```python
from build123d import *

# Parameters (mm, degrees)
CROQUIS1_R                = 1.5
SALIENTE_EXTRUIR2_DEPTH   = 3
SALIENTE_EXTRUIR2_2_DEPTH = 3
SALIENTE_EXTRUIR3_DEPTH   = 3
CROQUIS4_R                = 1.5
CORTAR_EXTRUIR2_DEPTH     = 3
SALIENTE_EXTRUIR4_START   = -3
CROQUIS5_R                = 1.5
SALIENTE_EXTRUIR4_DEPTH   = 3
SALIENTE_EXTRUIR5_DEPTH   = 15
CROQUIS7_R                = 1.5
CORTAR_EXTRUIR3_DEPTH     = 15
CROQUIS8_R                = 1.5
CORTAR_EXTRUIR4_DEPTH     = 15
CROQUIS9_R                = 1.5
CORTAR_EXTRUIR5_DEPTH     = 15
CROQUIS10_W               = 207.078994109
CROQUIS10_H               = 142.865408101
CORTAR_EXTRUIR6_DEPTH     = 20
SALIENTE_EXTRUIR6_DEPTH   = 3
CORTAR_EXTRUIR9_DEPTH     = 6
SALIENTE_EXTRUIR8_DEPTH   = 6
CROQUIS14_W               = 35.322230026
CROQUIS14_H               = 29.345994137
CORTAR_EXTRUIR10_DEPTH    = 3
CROQUIS15_W               = 36.043333432
CROQUIS15_H               = 18.319096506
CORTAR_EXTRUIR12_DEPTH    = 10
SALIENTE_EXTRUIR9_DEPTH   = 15
CROQUIS17_R               = 1.5
CORTAR_EXTRUIR14_DEPTH    = 30
CROQUIS18_R               = 1.5
CORTAR_EXTRUIR15_DEPTH    = 30


with BuildPart() as part:
    # Croquis1 → Saliente-Extruir2 (new body)
    with BuildSketch(Plane(origin=(0, 0, 0), x_dir=(1, 0, 0), z_dir=(0, 1, 0))):
        Polygon((35, 0), (65, 0), (167.530483272, -102.530483272), (161.873629023, -108.187337522), (61.686291501, -8), (35, -8), align=None)
        with Locations(Location((50, -4, 0), (0, 0, 270))):
            Circle(CROQUIS1_R, mode=Mode.SUBTRACT)
        with Locations(Location((159.045201898, -99.702056147, 0), (0, 0, 270))):
            Circle(CROQUIS1_R, mode=Mode.SUBTRACT)
        with Locations(Location((67.828427125, -8.485281374, 0), (0, 0, 270))):
            Circle(CROQUIS1_R, mode=Mode.SUBTRACT)
    extrude(amount=SALIENTE_EXTRUIR2_DEPTH)



with BuildPart() as body_2:
    # Croquis1 → Saliente-Extruir2 2 (new body)
    with BuildSketch(Plane(origin=(0, 0, 0), x_dir=(1, 0, 0), z_dir=(0, 1, 0))):
        Polygon((-35, 0), (-65, 0), (-167.530483272, -102.530483272), (-161.873629023, -108.187337522), (-61.686291501, -8), (-35, -8), align=None)
        with Locations(Location((-50, -4, 0), (0, 0, 270))):
            Circle(CROQUIS1_R, mode=Mode.SUBTRACT)
        with Locations(Location((-67.828427125, -8.485281374, 0), (0, 0, 270))):
            Circle(CROQUIS1_R, mode=Mode.SUBTRACT)
        with Locations(Location((-159.045201898, -99.702056147, 0), (0, 0, 270))):
            Circle(CROQUIS1_R, mode=Mode.SUBTRACT)
    extrude(amount=SALIENTE_EXTRUIR2_2_DEPTH)


with BuildPart() as part_1:
    add(part.part)

    add(body_2.part)  # Saliente-Extruir3 merges body 2
    # Croquis3 → Saliente-Extruir3 (add)
    with BuildSketch(Plane(origin=(0, 3, 0), x_dir=(1, 0, 0), z_dir=(0, 1, 0))):
        Polygon((-161.873629023, -108.187337522), (-159.752308679, -110.308657865), (-60.443650814, -11), (-35, -11), (-35, -8), (-61.686291501, -8), align=None)
        Polygon((35, -8), (61.686291501, -8), (161.873629023, -108.187337522), (159.752308679, -110.308657865), (60.443650814, -11), (35, -11), align=None)
    extrude(amount=-SALIENTE_EXTRUIR3_DEPTH)

    # Croquis4 → Cortar-Extruir2 (cut)
    with BuildSketch(Plane(origin=(0, 3, 0), x_dir=(1, 0, 0), z_dir=(0, 1, 0))):
        with Locations(Location((-50, -7.1, 0), (0, 0, 270))):
            Circle(CROQUIS4_R)
        with Locations(Location((-65.636396103, -10.677312396, 0), (0, 0, 270))):
            Circle(CROQUIS4_R)
        with Locations(Location((-156.853170876, -101.894087169, 0), (0, 0, 270))):
            Circle(CROQUIS4_R)
        with Locations(Location((50, -7.1, 0), (0, 0, 270))):
            Circle(CROQUIS4_R)
        with Locations(Location((65.636396103, -10.677312396, 0), (0, 0, 270))):
            Circle(CROQUIS4_R)
        with Locations(Location((156.853170876, -101.894087169, 0), (0, 0, 270))):
            Circle(CROQUIS4_R)
    extrude(amount=-CORTAR_EXTRUIR2_DEPTH, mode=Mode.SUBTRACT)

    # Croquis5 → Saliente-Extruir4 (add)
    with BuildSketch(Plane(origin=(0, 3, 0), x_dir=(1, 0, 0), z_dir=(0, 1, 0)).offset(SALIENTE_EXTRUIR4_START)):
        with Locations((-159.045201898, -99.702056147)):
            Circle(CROQUIS5_R)
        with Locations((-67.828427125, -8.485281374)):
            Circle(CROQUIS5_R)
        with Locations((-50, -4)):
            Circle(CROQUIS5_R)
        with Locations((50, -4)):
            Circle(CROQUIS5_R)
        with Locations((67.828427125, -8.485281374)):
            Circle(CROQUIS5_R)
        with Locations((159.045201898, -99.702056147)):
            Circle(CROQUIS5_R)
    extrude(amount=SALIENTE_EXTRUIR4_DEPTH)

    # Croquis6 → Saliente-Extruir5 (add)
    with BuildSketch(Plane(origin=(0, 0, 0), x_dir=(-1, 0, 0), z_dir=(0, -1, 0))):
        Polygon((167.530483272, -102.530483272), (65, 0), (35, 0), (35, -3), (63.757359313, -3), (165.409162928, -104.651803616), align=None)
        Polygon((-35, 0), (-35, -3), (-63.757359313, -3), (-165.409162928, -104.651803616), (-167.530483272, -102.530483272), (-65, 0), align=None)
    extrude(amount=SALIENTE_EXTRUIR5_DEPTH)

    # Croquis7 → Cortar-Extruir3 (cut)
    with BuildSketch(Plane(origin=(0, 0, 0), x_dir=(-1, 0, 0), z_dir=(0, 0, -1))):
        with Locations((50, -7.5)):
            Circle(CROQUIS7_R)
        with Locations((-50, -7.5)):
            Circle(CROQUIS7_R)
    extrude(amount=-CORTAR_EXTRUIR3_DEPTH, mode=Mode.SUBTRACT)

    # Croquis8 → Cortar-Extruir4 (cut)
    with BuildSketch(Plane(origin=(-32.5, 0, -32.5), x_dir=(-0.7071067811865476, 0, 0.7071067811865476), z_dir=(-0.7071067811865476, 0, -0.7071067811865476))):
        with Locations((182.961940777, -7.5)):
            Circle(CROQUIS8_R)
        with Locations((53.961940777, -7.5)):
            Circle(CROQUIS8_R)
    extrude(amount=-CORTAR_EXTRUIR4_DEPTH, mode=Mode.SUBTRACT)

    # Croquis9 → Cortar-Extruir5 (cut)
    with BuildSketch(Plane(origin=(32.5, 0, -32.5), x_dir=(-0.7071067811865476, 0, -0.7071067811865476), z_dir=(0.7071067811865476, 0, -0.7071067811865476))):
        with Locations((-182.961940777, -7.5)):
            Circle(CROQUIS9_R)
        with Locations((-53.961940777, -7.5)):
            Circle(CROQUIS9_R)
    extrude(amount=-CORTAR_EXTRUIR5_DEPTH, mode=Mode.SUBTRACT)

    # Croquis10 → Cortar-Extruir6 (cut)
    with BuildSketch(Plane(origin=(0, 3, 0), x_dir=(1, 0, 0), z_dir=(0, 1, 0))):
        with Locations((-138.539497055, -71.432704051)):
            Rectangle(CROQUIS10_W, CROQUIS10_H)
    extrude(amount=-CORTAR_EXTRUIR6_DEPTH, mode=Mode.SUBTRACT)

    # Croquis11 → Saliente-Extruir6 (add)
    with BuildSketch(Plane(origin=(0, 3, 0), x_dir=(1, 0, 0), z_dir=(0, 1, 0))):
        Polygon((65, 0), (35.287813482, 4.145596742), (33.767761344, -6.748871648), (59.828674856, -10.385024042), (60.443650814, -11), align=None)
    extrude(amount=SALIENTE_EXTRUIR6_DEPTH)

    # Croquis12 → Cortar-Extruir9 (cut)
    with BuildSketch(Plane(origin=(0, 6, 0), x_dir=(1, 0, 0), z_dir=(0, 1, 0))):
        Polygon((35, -6.920799909), (35, -11), (60.443650814, -11), (59.828674856, -10.385024042), align=None)
    extrude(amount=-CORTAR_EXTRUIR9_DEPTH, mode=Mode.SUBTRACT)

    # Croquis13 → Saliente-Extruir8 (add)
    with BuildSketch(Plane(origin=(0, 6, 0), x_dir=(1, 0, 0), z_dir=(0, 1, 0))):
        Polygon((35.287813482, 4.145596742), (33.767761344, -6.748871648), (59.828674856, -10.385024042), (60.443650814, -11), (65, 0), align=None)
    extrude(amount=-SALIENTE_EXTRUIR8_DEPTH)

    # Croquis14 → Cortar-Extruir10 (cut)
    with BuildSketch(Plane(origin=(0, 6, 0), x_dir=(1, 0, 0), z_dir=(0, 1, 0))):
        with Locations((49.859763615, -7.874178501)):
            Rectangle(CROQUIS14_W, CROQUIS14_H)
    extrude(amount=-CORTAR_EXTRUIR10_DEPTH, mode=Mode.SUBTRACT)

    # Croquis15 → Cortar-Extruir12 (cut)
    with BuildSketch(Plane(origin=(1.241209114, 0, -8.895953705), x_dir=(-0.9904062172531622, 0, -0.1381865580520849), z_dir=(0.1381865580520849, 0, -0.9904062172531622))):
        with Locations((-46.354737405, -9.159548253)):
            Rectangle(CROQUIS15_W, CROQUIS15_H)
    extrude(amount=-CORTAR_EXTRUIR12_DEPTH, mode=Mode.SUBTRACT)

    # Croquis16 → Saliente-Extruir9 (add)
    with BuildSketch(Plane(origin=(0, 0, 0), x_dir=(-1, 0, 0), z_dir=(0, -1, 0))):
        Polygon((-35.287813482, 4.145596742), (-65, 0), (-64.480524839, -3.723165526), (-63.589638597, -2.832279284), (-34.873253808, 1.17437809), align=None)
        Polygon((-66.286556106, -3.282217184), (-65, 0), (-64.480524839, -3.723165526), align=None)
    extrude(amount=SALIENTE_EXTRUIR9_DEPTH)

    # Croquis17 → Cortar-Extruir14 (cut)
    with BuildSketch(Plane(origin=(0, -15, 0), x_dir=(-1, 0, 0), z_dir=(0, -1, 0))):
        with Locations(Location((-56.0956257, -5.926391678, 0), (0, 0, 90))):
            Circle(CROQUIS17_R)
    extrude(amount=-CORTAR_EXTRUIR14_DEPTH, mode=Mode.SUBTRACT)

    # Croquis18 → Cortar-Extruir15 (cut)
    with BuildSketch(Plane(origin=(1.241209114, 0, -8.895953705), x_dir=(-0.9904062172531622, 0, -0.1381865580520849), z_dir=(0.1381865580520849, 0, -0.9904062172531622))):
        with Locations((-56.376404121, -4.1)):
            Circle(CROQUIS18_R)
    extrude(amount=-CORTAR_EXTRUIR15_DEPTH, mode=Mode.SUBTRACT)


solid = part_1.part
```
Geometry check sheet. Reference: the model listing, model coordinates, mm. A direction names the side the tool comes from. Coordinates: 2 decimals unless noted, no trailing zeros. Order: outer loops, then holes, each group sorted by start corner. A loop starts at its lowest first (then second) coordinate and runs counter-clockwise, first axis right, second up.
Q1. Thickness scan on probe 1 along Y at (x, z) = (125, 68.5); probe 2 along X at (y, z) = (-8.5, 10.5); probe 3 along X at (y, z) = (-2, 12). Record the ranges inside material, lowest first.
Reply:
probe 1: y = 0 to 3
probe 2: x = 71.26 to 75.5
probe 3: x = 72.76 to 77
Q2. Sectioned sample at B-B on z = 22.5. Record the cut outline in (x, y), and give its area (3 significant figures).
Reply:
outline: (71.94, 0) - (83.26, 0) - (83.26, -15) - (87.5, -15) - (87.5, 3) - (71.94, 3) - close
area: 110 mm2
Q3. Draft check along Z on faces 1 (the face through (49.432, -7.395, 0.857)), 2 (the face through (49.94, -5.87, -2.1)), 3 (the face through (161.67, -8.413, 98.761)). Enter one of: released by +Z, released by -Z, zero draft, split by the parting line, or undercut.
Reply:
face 1: released by +Z
face 2: released by -Z
face 3: undercut
Q4. Sectioned sample at C-C on x = 153. Record the cut outline in (y, z).
Reply:
outline: (-15, 88) - (3, 88) - (3, 103.56) - (0, 103.56) - (0, 92.24) - (-15, 92.24) - close
Q5. Depth check by flat-ended pin: pin 1 Ø6 at (x, y) = (96, -2.5) entering from +Z; pin 2 Ø6 at (x, z) = (111, 57.5) entering from -Y; pin 3 Ø6 at (x, y) = (76.5, -6.5) entering from +Z. Enter the tip coordinate at first touch or a pass-through.
Reply:
pin 1: stops at z = 48.21
pin 2: stops at y = 0
pin 3: stops at z = 18.74
Q6. Tool access check on faces 4 (the face through (106, -15, 42)), 5 (the face through (104, 0, 50)). Record the directions out of +Z, -Z, +X, -X, +Y, -Y that give a thin tool (end or side, any length) a straight path to the whole face; none if there is none.
Reply:
face 4: +Z, -Z, +X, -X, -Y
face 5: +Z, -X, -Y
Q7. Sectioned sample at A-A on y = -13. Record the cut outline in (x, z), and give its area (3 significant figures).
Reply:
outline: (34.87, -1.17) - (35.29, -4.15) - (65, 0) - (167.53, 102.53) - (165.41, 104.65) - (63.59, 2.83) - close
area: 522 mm2
